Autodesk Inventor part; units mm, degrees
ref_plane "YZ Plane" through (0, 0, 0) normal (1, 0, 0) x (0, 1, 0)
ref_plane "XZ Plane" through (0, 0, 0) normal (0, 1, 0) x (-1, 0, 0)
ref_plane "XY Plane" through (0, 0, 0) normal (0, 0, 1) x (1, 0, 0)
sketch "Sketch1" plane through (0, 0, 0) normal (0, 1, 0) x (-1, 0, 0)
  circle A0 centre (0, 0) radius 61
  circle A1 centre (0, 0) radius 58
  circle A2 centre (0, 0) radius 64
  dimension "d0" = 122
  dimension "d1" = 3
  dimension "d2" = 3
extrude "Extrusion1" add sketch "Sketch1" along normal blind 11 contours A0
extrude "Extrusion2" add sketch "Sketch1" along normal blind 3 contours A2
sketch "Sketch2" plane through (0, 3, 0) normal (0, 1, 0) x (1, 0, 0)
  circle A0 centre (-4.5, -61.8365) radius 1
  circle A1 centre (0, 0) radius 61
  circle A2 centre (0, 0) radius 63 construction
  circle A3 centre (4.5, -63.8416) radius 1
  dimension "d7" = 2
  dimension "d8" = 4.5
  dimension "d9" = 4.5
extrude "Extrusion3" cut sketch "Sketch2" against normal up to surface (3 mm away) contours A0 | A3
extrude "Extrusion4" add sketch "Sketch1" along normal blind 3 contours A1
sketch "Sketch3" plane through (0, 0, 0) normal (0, -1, 0) x (1, 0, 0)
  line L0 (64, -7.5) -> (44, -7.5)
  line L1 (44, -7.5) -> (44, 7.5)
  line L2 (44, 7.5) -> (64, 7.5)
  line L3 (64, 7.5) -> (64, -7.5)
  arc A0 (3.502, 63.9041) -> (5.4969, 63.7635) centre (0, 0) ccw
  point P0 (64, 0)
  dimension "d14" = 15
  dimension "d15" = 20
extrude "Extrusion5" cut sketch "Sketch3" against normal up to surface (11 mm away)
pattern_circular "Circular Pattern1" count 3 over 180 about axis through (0, -10, 0) along (0, 1, 0) of "Extrusion5"
fillet "Fillet1" radius 3 6 edges at (44, 1.5, 7.5) (44, 1.5, -7.5) (-44, 1.5, 7.5) (-44, 1.5, -7.5) (7.5, 1.5, -44) (-7.5, 1.5, -44)
properties part number "122mm-CoilForm_3DPrint"
Source: CAD feature listing. Evaluate the final solid. Frame: model axes, mm. A direction names the side the tool comes from. Coordinates: 2 decimals unless noted, no trailing zeros. Write each loop counter-clockwise with the first axis right and the second up, starting at its lowest first coordinate (ties: lowest second). Pieces come first, ordered by that corner, then holes. Notation, with made-up numbers: M 1,63.25 L 36,63.25 A8 cw 36,73.25 Z; hole C 66.25,65 d10. An arc over 180 degrees is marked long. Use a Markdown table: item, result.
1) Section B-B, the plane z = -51. Output: boundary loops of the cut face in (x, y).
Conclusion:
| item | result |
|---|---|
| outline | M -38.67,0 L -7.5,0 L -7.5,3 L -27.62,3 L -27.62,11 L -33.47,11 L -33.47,3 L -38.67,3 Z; M 7.5,0 L 38.67,0 L 38.67,3 L 33.47,3 L 33.47,11 L 27.62,11 L 27.62,3 L 7.5,3 Z |
2) First-contact query: pin 1 Ø12 at (x, z) = (-34, -23) entering from +Y; pin 2 Ø5.5 at (y, z) = (4, -53) entering from -X; pin 3 Ø3 at (y, z) = (1.5, -45.5) entering from +X; pin 4 Ø5 at (x, z) = (25.5, -23) entering from -Y. Flat tips, straight axial feed; report the tip coordinate or a pass-through.
Conclusion:
| item | result |
|---|---|
| pin 1 | stops at y = 3 |
| pin 2 | stops at x = -39.4 |
| pin 3 | stops at x = 46.48 |
| pin 4 | stops at y = 0 |
3) Reachability of faces 5 (the flat face through (44, 3, -44)), 6 (the cylindrical face through (-44.9, 1.52, 6.64)), 7 (the cylindrical face through (6.6, 1.52, -44.86)), 8 (the cylindrical face through (-43.531, 6.944, -42.732)), 9 (the flat face through (55, 2, -7.5)) from +Z, -Z, +X, -X, +Y, -Y: full face, straight path, thin tool, end or side. Return the list, or none.
Conclusion:
| item | result |
|---|---|
| face 5 | -Z, +X, +Y |
| face 6 | -X, +Y, -Y |
| face 7 | -Z, +Y, -Y |
| face 8 | -Z, -X, +Y |
| face 9 | +X, +Y, -Y |
4) Mould query, pull axis X, two halves, no side actions, for faces 1 (the cylindrical face through (44.83, 1.479, -45.676)), 2 (the flat face through (55, 2, 7.5)), 3 (the cylindrical face through (-41.39, 6.94, -40.63)), 4 (the flat face through (-44, 1, 0)). Classes: pulls with the +X half, pulls with the -X half, needs draft (parallel to the pull), parting line crosses it, or undercut.
Conclusion:
| item | result |
|---|---|
| face 1 | pulls with the +X half |
| face 2 | needs draft |
| face 3 | undercut |
| face 4 | pulls with the -X half |
5) Section A-A, the plane y = 6.5. Output: boundary loops of the cut face in (x, z).
Conclusion:
| item | result |
|---|---|
| outline | M -60.54,-7.5 A61 ccw -7.5,-60.54 L -7.5,-57.51 A58 cw -57.51,-7.5 Z; M -60.54,7.5 L -57.51,7.5 A58 cw 57.51,7.5 L 60.54,7.5 A61 ccw Z; M 7.5,-60.54 A61 ccw 60.54,-7.5 L 57.51,-7.5 A58 cw 7.5,-57.51 Z |
6) Section D-D, the plane z = 16. Output: boundary loops of the cut face in (x, y).
Conclusion:
| item | result |
|---|---|
| outline | M -61.97,0 L 61.97,0 L 61.97,3 L 58.86,3 L 58.86,11 L 55.75,11 L 55.75,3 L -55.75,3 L -55.75,11 L -58.86,11 L -58.86,3 L -61.97,3 Z |
7) Ray query, L1, parallel to Y at x = -42.5, z = 11; L2, parallel to Z at x = -8.5, y = 4.75; L3, parallel to X at y = 9, z = -31. Return the intervals inside material, ascending.
Conclusion:
| item | result |
|---|---|
| L1 | y = 0 to 3 |
| L2 | z = -60.4 to -57.37, 57.37 to 60.4 |
| L3 | x = -52.54 to -49.02, 49.02 to 52.54 |
8) Section C-C, the plane x = -27. Output: boundary loops of the cut face in (y, z), then the cut area to 3 significant figures.
Conclusion:
| item | result |
|---|---|
| outline | M 0,-58.03 L 3,-58.03 L 3,-54.7 L 11,-54.7 L 11,-51.33 L 3,-51.33 L 3,51.33 L 11,51.33 L 11,54.7 L 3,54.7 L 3,58.03 L 0,58.03 Z |
| area | 402 mm^2 |
